Design review of the part built by this model. Coordinates are the model's own, in mm. A direction names the side the tool comes from. Coordinates: 2 decimals unless noted, no trailing zeros. Loops run counter-clockwise (first coordinate to the right, second up) from the corner with the lowest first, then second, coordinate; pieces in that order, holes last. Notation, with made-up numbers: M 12.5,66 L 69.5,66 A12 cw 69.5,74 Z; hole C 75.25,-1 d8. An arc over 180 degrees is marked long. One line per item, written item: value.
```python
from build123d import *

# Parameters (mm, degrees)
HOLE_WIZARD_M5_1_D    = 4.2
M20X1_5_1_D           = 15
M20X1_5_1_CBORE_D     = 20
M20X1_5_1_CBORE_DEPTH = 13
CHAMFER_1_SIZE        = 0.5
CHAMFER_2_SIZE        = 1
FILLET_1_R            = 0.5


with BuildPart() as part:
    # 草图1 → 旋转1 (revolve)
    with BuildSketch(Plane(origin=(0, 0, 0), x_dir=(-1, 0, 0), z_dir=(0, 0, -1)), mode=Mode.PRIVATE) as revolve_1_sk:
        Polygon((-28, 0), (0, 0), (0, 22.55), (-12.5, 22.55), (-12.5, 20.85), (-11.95, 20.85), (-11.95, 19.5), (-12.5, 19.5), (-12.5, 6), (-13.5, 6), (-13.5, 5), (-28, 5), align=None)
    revolve(revolve_1_sk.sketch.rotate(Axis((0, 0, 0), (0, 1, 0)), 180), axis=Axis((0, 0, 0), (0, 1, 0)))

    # M5 螺纹孔1 (through all)
    with Locations(Plane(origin=(0, 0, 0), x_dir=(-1, 0, 0), z_dir=(0, -1, 0))):
        with Locations((0, -22), (-19.052558883, -11), (-19.052558883, 11), (0, 22), (19.052558883, 11), (19.052558883, -11)):
            Hole(HOLE_WIZARD_M5_1_D / 2)

    # M20x1.5 螺纹孔1 (through all)
    with Locations(Plane(origin=(0, 0, 0), x_dir=(-1, 0, 0), z_dir=(0, -1, 0))):
        with Locations((0, 0)):
            CounterBoreHole(M20X1_5_1_D / 2, M20X1_5_1_CBORE_D / 2, M20X1_5_1_CBORE_DEPTH)

    # 倒角1
    chamfer_1_edges = [part.edges().sort_by_distance(p)[0] for p in [
        (12.5, 22.55, 0),
    ]]
    chamfer(chamfer_1_edges, length=CHAMFER_1_SIZE)

    # 倒角2
    chamfer_2_edges = [part.edges().sort_by_distance(p)[0] for p in [
        (28, 0, 0),
        (10, 0, 0),
        (28, 5, 0),
    ]]
    chamfer(chamfer_2_edges, length=CHAMFER_2_SIZE)

    # 圆角1
    fillet_1_edges = [part.edges().sort_by_distance(p)[0] for p in [
        (13.5, 5, 0),
    ]]
    fillet(fillet_1_edges, radius=FILLET_1_R)


solid = part.part
```
(1) Mouldability with a two-part tool opening along X and no side actions: class faces 4 (the flat face through (-12, 0, 0)), 5 (the cylindrical face through (-7.493, 17.842, -0.33)), 6 (the cylindrical face through (-6.42, 20.17, 10.08)) as released by +X, released by -X, zero draft, split by the parting line, or undercut.
Reply:
face 4: zero draft
face 5: undercut
face 6: split by the parting line
(2) Insertion check: pin 1 (5 mm diameter, centred on x = 19.05, z = 11, fed in from +Y); pin 2 (12 mm diameter, centred on y = 20, z = -10.5, fed in from +X); pin 3 (5 mm diameter, centred on y = 17, z = 13, fed in from +X); pin 4 (12 mm diameter, centred on x = 2.5, z = -6, fed in from -Y). Each pin has a flat end and moves straight along its axis. Give the tip position at first contact, or say it passes through.
Reply:
pin 1: stops at y = 5
pin 2: stops at x = 11.65
pin 3: stops at x = 6.78
pin 4: stops at y = 0
(3) We need section B-B on x = 0. State how many separate pieces and enclosed holes the cut face has, then the cut area to 3 significant figures.
Reply:
separate pieces: 4
enclosed holes: 0
area: 271 mm2
(4) Tool access review of faces 1 (the flat face through (12, 5, -12)), 2 (the cylindrical face through (1.13, 2.53, 20.23)), 3 (the flat face through (-4, 13, -7)): name each direction out of +Z, -Z, +X, -X, +Y, -Y from which nothing blocks a thin tool from reaching the whole face with its end or side.
Reply:
face 1: +Y
face 2: +Y, -Y
face 3: -Y
(5) To check wall thickness, follow line 1 along Z through (x, y) = (0, 1); line 2 along Z through (x, y) = (17.5, 4.5); line 3 along Y through (x, z) = (-12.5, -10.5). State the ranges of each line that lie inside material, in increasing order. Write a range as [from, to].
Reply:
line 1: z = [-28, -24.1], [-19.9, -10], [10, 19.9], [24.1, 28]
line 2: z = [-21.21, -12.41], [-9.59, 9.59], [12.41, 21.21]
line 3: y = [0, 5]
(6) We need section A-A on y = 2.25. State the section outline as (x, z) points, then the cut area to 3 significant figures.
Reply:
outline: C 0,0 d56; hole C -19.05,-11 d4.2; hole C -19.05,11 d4.2; hole C 0,0 d20; hole C 0,-22 d4.2; hole C 0,22 d4.2; hole C 19.05,-11 d4.2; hole C 19.05,11 d4.2
area: 2,070 mm2
(7) We need section C-C on y = 14.5. State the section outline as (x, z) points, then the cut area to 3 significant figures.
Reply:
outline: C 0,0 d25; hole C 0,0 d15
area: 314 mm2
